from build123d import *

# Parameters (mm, degrees)
F0_W     = 50.8
F0_H     = 31.75
F1_DEPTH = 50.8
F3_DEPTH = 25.4
F5_DEPTH = 25.4


with BuildPart() as f1:
    # F0 (on Front) → F1 (new body)
    with BuildSketch(Plane.XZ):
        with Locations((25.4, 15.875)):
            Rectangle(F0_W, F0_H)
    extrude(amount=F1_DEPTH)

    # F2 (on face) → F3 (cut)
    with BuildSketch(Plane.XZ.offset(50.8)):
        Polygon((50.8, 31.75), (18.300158903, 31.75), (35.8910150826, 0), (50.8, 0), align=None)
    extrude(amount=-F3_DEPTH, mode=Mode.SUBTRACT)

    # F4 (on face) → F5 (cut)
    with BuildSketch(Plane.XZ.offset(25.4)):
        Polygon((18.300158903, 31.75), (28.4925211666, 13.3536525702), (50.8, 13.3536525702), (50.8, 31.75), align=None)
    extrude(amount=-F5_DEPTH, mode=Mode.SUBTRACT)


solid = f1.part
Geometry check sheet. Reference: the model listing, model coordinates, mm. A direction names the side the tool comes from. Give positions to 0.01 mm unless a question says otherwise; leave off trailing zeros. Order: outer loops, then holes, each group sorted by start corner. A loop starts at its lowest first (then second) coordinate and runs counter-clockwise, first axis right, second up.
1. Depth check by flat-ended pin: pin 1 (4 mm diameter, centred on x = 35.5, z = 7, fed in from -Y); pin 2 (6.5 mm diameter, centred on x = 34.5, y = -10, fed in from +Z); pin 3 (3 mm diameter, centred on y = -22.5, z = 27, fed in from +X). Enter the tip coordinate at first touch or a pass-through.
Completed:
pin 1: stops at y = -25.4
pin 2: stops at z = 13.35
pin 3: stops at x = 21.76
2. Sectioned sample at C-C (x = 26.5). Record the boundary of the cut face in (y, z), then the cut area to 3 significant figures.
Completed:
outline: (-50.8, 0) - (0, 0) - (0, 16.95) - (-50.8, 16.95) - close
area: 861 mm2
3. Scan lines: line 1 (Z direction, x = 30, y = -22); line 2 (Y direction, x = 33, z = 13); line 3 (X direction, y = -49, z = 29.5). Record each from-to range of solid material in increasing order.
Completed:
line 1: z = 0 to 13.35
line 2: y = -25.4 to 0
line 3: x = 0 to 19.55
4. Sectioned sample at B-B (z = 14). Record the boundary of the cut face in (x, y).
Completed:
outline: (0, -50.8) - (28.13, -50.8) - (28.13, 0) - (0, 0) - close
5. Sectioned sample at A-A (y = -3.5). Record the boundary of the cut face in (x, z), then the cut area to 3 significant figures.
Completed:
outline: (0, 0) - (50.8, 0) - (50.8, 13.35) - (28.49, 13.35) - (18.3, 31.75) - (0, 31.75) - close
area: 1,110 mm2
6. Access from +Z, -Z, +X, -X, +Y, -Y to the whole of each face (thin tool, end or side, straight path). Record for faces 1 (the face through (39, -13, 13.354)), 2 (the face through (42, -25.4, 7)), 3 (the face through (19, -25, 0)).
Completed:
face 1: +Z, +X, +Y, -Y
face 2: +Z, +X, -Y
face 3: -Z, +X, -X, +Y, -Y
7. Sectioned sample at D-D (z = 7). Record the boundary of the cut face in (x, y).
Completed:
outline: (0, -50.8) - (32.01, -50.8) - (32.01, -25.4) - (50.8, -25.4) - (50.8, 0) - (0, 0) - close
